The listing builds one solid part. Answer for the finished solid, in the listing's coordinates (mm). A direction names the side the tool comes from. Give positions to 0.01 mm unless a question says otherwise; leave off trailing zeros. Loops run counter-clockwise (first coordinate to the right, second up) from the corner with the lowest first, then second, coordinate; pieces in that order, holes last. Notation, with made-up numbers: (40.5, 74.5) - (72.5, 74.5) arc R30 cw to (72.5, 96.5) - close; hole circle Ø3 at (-16, 58). An arc over 180 degrees is marked (long way). One line per item, written item: value. Start each with the question number.
from build123d import *

# Parameters (mm, degrees)
SKETCH1_W           = 1.5113
SKETCH1_H           = 1.1938
SKETCH1_R           = 3.7338
SKETCH1_R_2         = 0.9525
BOSS_EXTRUDE1_DEPTH = 1.5875


with BuildPart() as part:
    # Sketch1 → Boss-Extrude1 (new body)
    with BuildSketch(Plane(origin=(0, 0, 0), x_dir=(0, 0, -1), z_dir=(1, 0, 0))):
        with BuildLine():
            Line((82.296, -12.181036366), (82.296, -6.2738))
            Line((82.296, -6.2738), (83.8708, -6.2738))
            ThreePointArc((83.8708, -6.2738), (87.402991636, -2.741608364), (83.8708, 0.790583272))
            Line((83.8708, 0.790583272), (82.296, 0.893791599))
            Line((82.296, 0.893791599), (82.296, 6.868963634))
            Line((82.296, 6.868963634), (83.8708, 6.868963634))
            Line((83.8708, 6.868963634), (83.8708, 8.900963634))
            Line((83.8708, 8.900963634), (80.264, 8.900963634))
            Line((80.264, 8.900963634), (62.185099246, 2.211808127))
            Line((62.185099246, 2.211808127), (0.410288477, 6.260369782))
            ThreePointArc((0.410288477, 6.260369782), (-6.270441547, 0.205254114), (0, -6.2738))
            Line((0, -6.2738), (62.185099246, -6.2738))
            Line((62.185099246, -6.2738), (80.264, -14.721036366))
            Line((80.264, -14.721036366), (83.8708, -14.721036366))
            Line((83.8708, -14.721036366), (83.8708, -12.181036366))
            Line((83.8708, -12.181036366), (82.296, -12.181036366))
        make_face()
        Polygon((39.325099246, 1.800906775), (62.185099246, 0.302721378), (62.185099246, -4.3688), (39.325099246, -4.3688), align=None, mode=Mode.SUBTRACT)
        Polygon((64.471099246, 0.152902838), (80.264, -0.882123115), (80.264, -4.3688), (64.471099246, -4.3688), align=None, mode=Mode.SUBTRACT)
        Polygon((66.3852906, -6.2738), (80.264, -6.2738), (80.264, -12.758527161), align=None, mode=Mode.SUBTRACT)
        with Locations((4.55295, -2.921)):
            Rectangle(SKETCH1_W, SKETCH1_H, mode=Mode.SUBTRACT)
        Circle(SKETCH1_R, mode=Mode.SUBTRACT)
        with BuildLine():
            Line((4.778751005, 4.064985273), (37.420099246, 1.925755558))
            Line((37.420099246, 1.925755558), (37.420099246, -4.3688))
            Line((37.420099246, -4.3688), (6.2738, -4.3688))
            Line((6.2738, -4.3688), (6.2738, 0))
            ThreePointArc((6.2738, 0), (5.888187094, 2.165599038), (4.778751005, 4.064985273))
        make_face(mode=Mode.SUBTRACT)
        Polygon((80.264, 1.026963634), (66.848818814, 1.906159984), (80.264, 6.869748995), align=None, mode=Mode.SUBTRACT)
        with Locations((84.8233, -2.741608364)):
            Circle(SKETCH1_R_2, mode=Mode.SUBTRACT)
    extrude(amount=BOSS_EXTRUDE1_DEPTH)


solid = part.part
1. A cutting plane is placed at C-C (x = 0.5). Give the number of separate pieces and of enclosed holes in the cut face, plus the area to 3 significant figures.
2. A cutting plane is placed at B-B (z = -68.5). Determine the outline of the cut face in (x, y).
3. For faces 4 (the flat face through (0.78, 0.84, -83.09)), 5 (the flat face through (1, -1, -37.42)), 6 (the flat face through (0.783, 4.208, -31.73)), 7 (the flat face through (1, -6.274, -31)), determine the directions among +Z, -Z, +X, -X, +Y, -Y from which every point of the face is accessible in a straight line to the end or side of a thin tool.
4. Flat-ended cylindrical pins translate along their axes: pin 1 (0.5 mm diameter, centred on x = 0.5, y = 4, fed in from +Z); pin 2 (10 mm diameter, centred on y = 3.5, z = -25, fed in from -X); pin 3 (0.8 mm diameter, centred on x = 0.5, y = -14, fed in from -Z); pin 4 (0.6 mm diameter, centred on x = 0.5, y = -2.5, fed in from +Z). Find the tip coordinate at first contact, or state that the pin passes through.
5. Find the intervals of material crossed by L1, parallel to Z at x = 1.3, y = -7.75; L2, parallel to Y at x = 0.7, z = -32.5; L3, parallel to Z at x = 0.6, y = -7.5, in increasing order. Write a range as [from, to].
6. Determine the mould class of faces 1 (the flat face through (1, -4.369, -51)), 2 (the flat face through (1, -13, -83.871)), 3 (the flat face through (0.78, -10.44, -71.1)) for opening direction Z: released by +Z, released by -Z, zero draft, split by the parting line, or undercut.
7. A cutting plane is placed at A-A (z = -9.5). Determine the outline of the cut face in (x, y), plus the area to 3 significant figures.
Results below:
1. separate pieces: 1
1. enclosed holes: 8
1. area: 543 mm^2
2. outline: (0, -9.22) - (1.59, -9.22) - (1.59, -7.26) - (0, -7.26) - close; (0, -6.27) - (1.59, -6.27) - (1.59, -4.37) - (0, -4.37) - close; (0, -0.11) - (1.59, -0.11) - (1.59, 1.8) - (0, 1.8) - close; (0, 2.52) - (1.59, 2.52) - (1.59, 4.55) - (0, 4.55) - close
3. face 4: -Z, +X, -X
3. face 5: +X, -X
3. face 6: +X, -X, +Y
3. face 7: +Z, +X, -X, -Y
4. pin 1: stops at z = 5.03
4. pin 2: stops at x = 0
4. pin 3: stops at z = -83.87
4. pin 4: stops at z = 5.88
5. L1: z = [-82.3, -80.26], [-69.54, -65.34]
5. L2: y = [-6.27, -4.37], [2.25, 4.16]
5. L3: z = [-82.3, -80.26], [-69.01, -64.81]
6. face 1: undercut
6. face 2: released by -Z
6. face 3: released by +Z
7. outline: (0, -6.27) - (1.59, -6.27) - (1.59, -4.37) - (0, -4.37) - close; (0, 3.76) - (1.59, 3.76) - (1.59, 5.66) - (0, 5.66) - close
7. area: 6.05 mm^2
